Verification items for the finished model (mm, model axes). A direction names the side the tool comes from. Give positions to 0.01 mm unless a question says otherwise; leave off trailing zeros. Order: outer loops, then holes, each group sorted by start corner. A loop starts at its lowest first (then second) coordinate and runs counter-clockwise, first axis right, second up.
(1) Mould release check, pull along Y, two halves, no side actions. Record for faces 1 (the face through (4, -10.65, 6)), 2 (the face through (4, -5, 5.407)), 3 (the face through (3, 0, 35)), 4 (the face through (4, -1, 0)): pulls with the +Y half, pulls with the -Y half, needs draft (parallel to the pull), parting line crosses it, or undercut.
(2) Access from +Z, -Z, +X, -X, +Y, -Y to the whole of each face (thin tool, end or side, straight path). Record for faces 5 (the face through (-4, -1, 59.643)), 6 (the face through (5.905, -7, 4)), 7 (the face through (3.92, -9.34, 7.12)), 8 (the face through (1.873, -7, 4)), 9 (the face through (4, -5, 0.494)).
(3) Sectioned sample at B-B on z = 16. Record the cut outline in (x, y).
(4) Gauge pin test, flat ends, axial feed: pin 1 (5 mm diameter, centred on x = 0, y = -9, fed in from -Z); pin 2 (1.5 mm diameter, centred on x = -2, y = -2, fed in from -Z); pin 3 (2.5 mm diameter, centred on y = -8.5, z = 2.5, fed in from +X). Record the tip position at first contact, or that the pin passes through.
(5) Sectioned sample at C-C on x = -4.25. Record the cut outline in (y, z), plus the area to 3 significant figures.
(6) Sectioned sample at A-A on y = -1. Record the cut outline in (x, z).
(7) Scan lines: L1, parallel to Z at x = 4.5, y = -4.5; L2, parallel to Y at x = 5.5, z = 9.5; L3, parallel to X at y = -2.5, z = 48. Record each from-to range of solid material in increasing order.
```python
from build123d import *

# Parameters (mm, degrees)
F1_DEPTH = 3
F2_W     = 4.032329
F2_H     = 4.912953
F3_DEPTH = 5
F4_W     = 4.032329
F4_H     = 4.912953


with BuildPart() as f1:
    # F0 (on Front) → F1 (new body)
    with BuildSketch(Plane.XZ):
        Polygon((1.371463, 67.128956), (1.371463, 0), (6.371463, 0), (6.371463, 70), (1.371463, 70), (-7.018532, 70), (-5.238707, 59.643164), (-2.930099, 59.643164), (-3.16445, 67.128956), align=None)
    extrude(amount=F1_DEPTH)

    # F2 (on face) → F3 (join)
    with BuildSketch(Plane.XZ.offset(3)):
        with Locations((3.889312, 2.950882)):
            Rectangle(F2_W, F2_H)
    extrude(amount=F3_DEPTH)

    # F6: sweep along a path in F5
    with BuildLine(Plane.YZ.offset(5.905477)) as f6_path:
        Line((-8, 5.407359), (-10.649814, 8.793468))
    # F4 (on face) → F6 (sweep)
    with BuildSketch(Plane.XZ.offset(8)):
        with Locations((3.889312, 2.950882)):
            Rectangle(F4_W, F4_H)
    sweep(path=f6_path.line)


solid = f1.part
```
Ans:
1. face 1: pulls with the -Y half
1. face 2: undercut
1. face 3: pulls with the +Y half
1. face 4: needs draft
2. face 5: -Z, -X, +Y, -Y
2. face 6: +Z, -Z, +X, -Y
2. face 7: +Z, +X, -X
2. face 8: +Z, -Z, -X, -Y
2. face 9: -Z, +X, -X, -Y
3. outline: (1.37, -3) - (6.37, -3) - (6.37, 0) - (1.37, 0) - close
4. pin 1: stops at z = 0.49
4. pin 2: stops at z = 67.13
4. pin 3: stops at x = 5.91
5. outline: (-3, 59.64) - (0, 59.64) - (0, 70) - (-3, 70) - close
5. area: 31.1 mm2
6. outline: (-7.02, 70) - (-5.24, 59.64) - (-2.93, 59.64) - (-3.16, 67.13) - (1.37, 67.13) - (1.37, 0) - (6.37, 0) - (6.37, 70) - close
7. L1: z = 0.49 to 5.41
7. L2: y = -3 to 0
7. L3: x = 1.37 to 6.37
